For this review, take the finished solid that the model builds, in its own axes (mm). Face numbers are marked on the shaded views. A direction names the side the tool comes from. Coordinates: 2 decimals unless noted, no trailing zeros. Loops run counter-clockwise (first coordinate to the right, second up) from the corner with the lowest first, then second, coordinate; pieces in that order, holes last. Notation, with made-up numbers: (68, 76.25) -> (123, 76.25) arc R30 ccw to (123, 107.25) -> close; hole circle Ø6 at (-15.5, 56.5). An arc over 180 degrees is marked (long way). One line per item, written item: value.
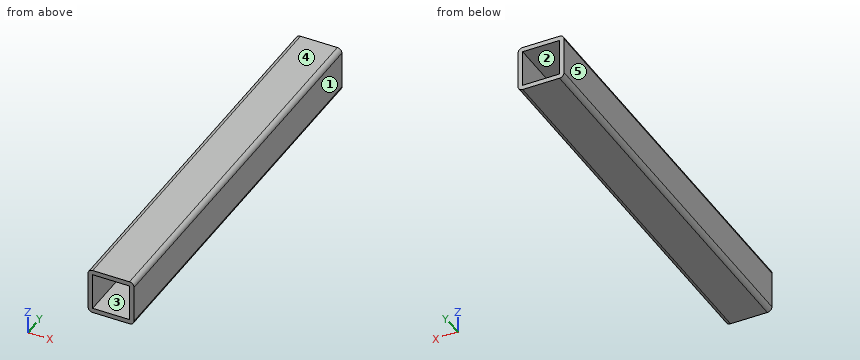
from build123d import *

# Parameters (mm, degrees)
CROQUIS1_W              = 24
CROQUIS1_H              = 24
SALIENTE_EXTRUIR1_DEPTH = 259.715457153


with BuildPart() as part:
    # Croquis1 → Saliente-Extruir1 (new body)
    with BuildSketch(Plane(origin=(0, 647.649993896, 0), x_dir=(1, 0, 0), z_dir=(0, 1, 0))):
        with BuildLine():
            Line((-12, 50.120137415), (12, 50.120137415))
            ThreePointArc((12, 50.120137415), (14.121320344, 50.998817072), (15, 53.120137415))
            Line((15, 53.120137415), (15, 77.120137415))
            ThreePointArc((15, 77.120137415), (14.121320344, 79.241457759), (12, 80.120137415))
            Line((12, 80.120137415), (-12, 80.120137415))
            ThreePointArc((-12, 80.120137415), (-14.121320344, 79.241457759), (-15, 77.120137415))
            Line((-15, 77.120137415), (-15, 53.120137415))
            ThreePointArc((-15, 53.120137415), (-14.121320344, 50.998817072), (-12, 50.120137415))
        make_face()
        with Locations((0, 65.120137415)):
            Rectangle(CROQUIS1_W, CROQUIS1_H, mode=Mode.SUBTRACT)
    extrude(amount=-SALIENTE_EXTRUIR1_DEPTH)


solid = part.part
1. Take a section at C-C, the plane x = -7.5. Give the boundary of the cut face in (y, z).
Return value:
outline: (387.93, -80.12) -> (647.65, -80.12) -> (647.65, -77.12) -> (387.93, -77.12) -> close; (387.93, -53.12) -> (647.65, -53.12) -> (647.65, -50.12) -> (387.93, -50.12) -> close
2. For the marked faces 1 and 2, list the 3-axis set-ups (+Z, -Z, +X, -X, +Y, -Y) from which the entire face can be reached by the end or side of a thin tool; tool diameter is ignored.
Return value:
face 1: +Z, -Z, +X, +Y, -Y
face 2: +Y, -Y
3. Take a section at A-A, the plane y = 576. Give the boundary of the cut face in (x, z), and give its area (3 significant figures).
Return value:
outline: (-15, -77.12) arc R3 ccw to (-12, -80.12) -> (12, -80.12) arc R3 ccw to (15, -77.12) -> (15, -53.12) arc R3 ccw to (12, -50.12) -> (-12, -50.12) arc R3 ccw to (-15, -53.12) -> close; hole (-12, -77.12) -> (12, -77.12) -> (12, -53.12) -> (-12, -53.12) -> close
area: 316 mm2
4. The part is to be moulded in two halves that separate along X. For the marked faces 3, 4 and 5, say which applies: pulls with the +X half, pulls with the -X half, needs draft (parallel to the pull), parting line crosses it, or undercut.
Return value:
face 3: undercut
face 4: needs draft
face 5: pulls with the -X half
5. To check wall thickness, follow probe 1 along Z at (x, y) = (-3, 492.5); probe 2 along X at (y, z) = (434, -65.5); probe 3 along X at (y, z) = (604, -77.25). State the ranges of each line that lie inside material, in increasing order. Write a range as from..to.
Return value:
probe 1: z = -80.12..-77.12, -53.12..-50.12
probe 2: x = -15..-12, 12..15
probe 3: x = -15..15
6. Take a section at B-B, the plane z = -59.25. Give the boundary of the cut face in (x, y).
Return value:
outline: (-15, 387.93) -> (-12, 387.93) -> (-12, 647.65) -> (-15, 647.65) -> close; (12, 387.93) -> (15, 387.93) -> (15, 647.65) -> (12, 647.65) -> close
